from build123d import *

# Parameters (mm, degrees)
BOSS_EXTRUDE1_DEPTH      = 32
SKETCH2_R                = 2
CUT_EXTRUDE1_DEPTH       = 35.869794274
LPATTERN1_COUNT          = 3
LPATTERN1_PITCH          = 8
BOSS_EXTRUDE2_DEPTH      = 9
BOSS_EXTRUDE2_DEPTH_BACK = 9
SKETCH3_W                = 32
SKETCH3_H                = 2
BOSS_EXTRUDE3_DEPTH      = 48
BOSS_EXTRUDE3_DEPTH_BACK = 48
SKETCH4_W                = 32
SKETCH4_H                = 3
SKETCH5_R                = 2.5
CUT_EXTRUDE2_DEPTH       = 10


with BuildPart() as part:
    # Sketch1 → Boss-Extrude1 (new body)
    with BuildSketch(Plane.XY):
        Polygon((9, 0), (-9, 0), (-11.309401077, 4), (-9, 8), (9, 8), (11.309401077, 4), align=None)
    extrude(amount=BOSS_EXTRUDE1_DEPTH)

    # Sketch2 → Cut-Extrude1 (cut, symmetric)
    with BuildSketch(Plane(origin=(0, 0, 0), x_dir=(0, 0, -1), z_dir=(1, 0, 0))):
        with Locations((-24, 4)):
            Circle(SKETCH2_R)
    cut_extrude1 = extrude(amount=CUT_EXTRUDE1_DEPTH, both=True, mode=Mode.SUBTRACT)

    # LPattern1: Cut-Extrude1 ×3
    with Locations(*[(0, 0, -i * LPATTERN1_PITCH) for i in range(1, LPATTERN1_COUNT)]):
        add(cut_extrude1, mode=Mode.SUBTRACT)

    # Sketch3 → Boss-Extrude2 (add, two sides: drawn at the far end of the back side and taken through both)
    with BuildSketch(Plane(origin=(0, 0, 0), x_dir=(0, 0, -1), z_dir=(1, 0, 0)).offset(-BOSS_EXTRUDE2_DEPTH_BACK)):
        with Locations((-16, 9)):
            Rectangle(SKETCH3_W, SKETCH3_H)
    extrude(amount=BOSS_EXTRUDE2_DEPTH + BOSS_EXTRUDE2_DEPTH_BACK)

    # Sketch4 → Boss-Extrude3 (add, two sides: drawn at the far end of the back side and taken through both)
    with BuildSketch(Plane(origin=(0, 0, 0), x_dir=(0, 0, -1), z_dir=(1, 0, 0)).offset(-BOSS_EXTRUDE3_DEPTH_BACK)):
        with Locations((-16, 11.5)):
            Rectangle(SKETCH4_W, SKETCH4_H)
    extrude(amount=BOSS_EXTRUDE3_DEPTH + BOSS_EXTRUDE3_DEPTH_BACK)

    # Sketch5 → Cut-Extrude2 (cut)
    with BuildSketch(Plane(origin=(0, 13, 0), x_dir=(1, 0, 0), z_dir=(0, 1, 0))):
        with Locations(Location((-37.55, -16, 0), (0, 0, 270))):
            Circle(SKETCH5_R)
        with Locations(Location((37.55, -16, 0), (0, 0, 270))):
            Circle(SKETCH5_R)
    extrude(amount=-CUT_EXTRUDE2_DEPTH, mode=Mode.SUBTRACT)


solid = part.part
Check sheet for the modelled part. Datum: model origin and axes. Units: mm. A direction names the side the tool comes from. Round coordinates to 2 decimals unless told otherwise and drop trailing zeros. Write each loop counter-clockwise with the first axis right and the second up, starting at its lowest first coordinate (ties: lowest second). Pieces come first, ordered by that corner, then holes. Notation, with made-up numbers: (35.5, 46.25) - (83.5, 46.25) arc R10 cw to (83.5, 51.25) - close; hole circle Ø8 at (39, 20). An arc over 180 degrees is marked (long way). Return JSON: item names as keys, results as strings.
Q1. Depth check by flat-ended pin: P1, Ø16, axis at x = 24, z = 18.5, coming from the -Y side; P2, Ø4.5, axis at x = -37.55, z = 16, coming from the -Y side; P3, Ø5, axis at y = 4, z = 24, coming from the +X side; P4, Ø1, axis at y = 9, z = 18, coming from the -X side. Enter the tip coordinate at first touch or a pass-through.
Returned:
{"P1": "stops at y = 10", "P2": "passes through", "P3": "stops at x = 11.31", "P4": "stops at x = -9"}
Q2. Cross-section at B-B (z = 7.5). Record the boundary of the cut face in (x, y).
Returned:
{"outline": "(-48, 10) - (-9, 10) - (-9, 8) - (-10.19, 5.94) - (10.19, 5.94) - (9, 8) - (9, 10) - (48, 10) - (48, 13) - (-48, 13) - close; (-10.19, 2.06) - (-9, 0) - (9, 0) - (10.19, 2.06) - close"}
Q3. Cross-section at A-A (x = -37.55). Record the boundary of the cut face in (y, z), then the cut area to 3 significant figures.
Returned:
{"outline": "(10, 0) - (13, 0) - (13, 13.5) - (10, 13.5) - close; (10, 18.5) - (13, 18.5) - (13, 32) - (10, 32) - close", "area": "81.0 mm²"}
Q4. Cross-section at D-D (z = 20.5). Record the boundary of the cut face in (x, y).
Returned:
{"outline": "(-48, 10) - (-9, 10) - (-9, 8) - (-11.31, 4) - (-9, 0) - (9, 0) - (11.31, 4) - (9, 8) - (9, 10) - (48, 10) - (48, 13) - (-48, 13) - close"}
Q5. Access from +Z, -Z, +X, -X, +Y, -Y to the whole of each face (thin tool, end or side, straight path). Record for faces 4 (the flat face through (9, 9, 16)), 5 (the cylindrical face through (0.158, 4.601, 6.092)), 6 (the flat face through (-9.91, 6.42, 15.78)).
Returned:
{"face 4": "+Z, -Z, +X", "face 5": "+X, -X", "face 6": "+Z, -Z, -X"}
Q6. Draft check along Z on faces 1 (the flat face through (0, 9, 32)), 2 (the cylindrical face through (35.1, 11.5, 15.5)), 3 (the flat face through (0, 0, 16)). Enter one of: released by +Z, released by -Z, zero draft, split by the parting line, or undercut.
Returned:
{"face 1": "released by +Z", "face 2": "undercut", "face 3": "zero draft"}
Q7. Scan lines: L1, parallel to X at y = 12.1, z = 16; L2, parallel to Z at x = -2.5, y = 4; L3, parallel to Y at x = 5.75, z = 8. Record each from-to range of solid material in increasing order. Write a range as from..to.
Returned:
{"L1": "x = -48..-40.05, -35.05..35.05, 40.05..48", "L2": "z = 0..6, 10..14, 18..22, 26..32", "L3": "y = 0..2, 6..13"}
Q8. Cross-section at C-C (x = -2.5). Record the boundary of the cut face in (y, z).
Returned:
{"outline": "(0, 0) - (13, 0) - (13, 32) - (0, 32) - close; hole circle Ø4 at (4, 8); hole circle Ø4 at (4, 16); hole circle Ø4 at (4, 24)"}
